Geometry check sheet. Reference: the model listing, model coordinates, mm. A direction names the side the tool comes from. Round coordinates to 2 decimals unless told otherwise and drop trailing zeros. Write each loop counter-clockwise with the first axis right and the second up, starting at its lowest first coordinate (ties: lowest second). Pieces come first, ordered by that corner, then holes.
Item 1: Access from +Z, -Z, +X, -X, +Y, -Y to the whole of each face (thin tool, end or side, straight path). Record for faces 4 (the face through (13.53, -17.05, 0.04)), 5 (the face through (8, 20, 0)), 6 (the face through (-8, 20, 0)).
Item 2: Depth check by flat-ended pin: P1, Ø1.5, axis at y = 23.5, z = -1, coming from the +X side; P2, Ø1, axis at y = -9.5, z = -1.5, coming from the +X side; P3, Ø19, axis at x = 0, y = 0, coming from the -Z side; P4, Ø22, axis at x = 3.5, y = -3.5, coming from the -Z side. Enter the tip coordinate at first touch or a pass-through.
Item 3: Cross-section at D-D (x = -19). Enter the section's corners in (y, z), then the cut area to 3 significant figures.
Item 4: Scan lines: probe 1 along Y at (x, z) = (0, 0); probe 2 along X at (y, z) = (27.5, -0.85); probe 3 along Z at (x, y) = (-0.5, 9). Record each from-to range of solid material in increasing order.
Item 5: Cross-section at C-C (y = 25). Enter the section's corners in (x, z), then the cut area to 3 significant figures.
Item 6: Cross-section at A-A (x = 0). Enter the section's corners in (y, z).
Item 7: Draft check along Z on faces 1 (the face through (-7, 10, -2.5)), 2 (the face through (13.04, 7.41, 0.04)), 3 (the face through (0, -7, 1.5)). Enter one of: pulls with the +Z half, pulls with the -Z half, needs draft (parallel to the pull), parting line crosses it, or undercut.
Item 8: Cross-section at B-B (z = -0.75). Enter the section's corners in (x, y).
from build123d import *

# Parameters (mm, degrees)
F0_R        = 10
F1_DEPTH    = 2.5
F0_R_2      = 6
F2_DEPTH    = 1.5
F3_T1_DEPTH = 15


# Not quite as in the source:
# - a fillet or chamfer that OpenCascade refuses, or shapes differently, is made with other operations: its cross-section is extruded or revolved along the edge and cut away or added


with BuildPart() as f1:
    # F0 (on Top) → F1 (new body, symmetric)
    with BuildSketch(Plane.XY):
        with BuildLine():
            Line((25.9807621135, -15), (29.9807621135, -8.0717967697))
            Line((29.9807621135, -8.0717967697), (14.9886304879, 0.5839144601))
            ThreePointArc((14.9886304879, 0.5839144601), (12.9903810568, 7.5), (8, 12.6885775404))
            Line((8, 12.6885775404), (8, 30))
            Line((8, 30), (-8, 30))
            Line((-8, 30), (-8, 12.6885775404))
            ThreePointArc((-8, 12.6885775404), (-12.9903810568, 7.5), (-14.9886304879, 0.5839144601))
            Line((-14.9886304879, 0.5839144601), (-27.4269246123, -6.5973380009))
            Line((-27.4269246123, -6.5973380009), (-29.9807621135, -8.0717967697))
            Line((-29.9807621135, -8.0717967697), (-21.9807621135, -21.9282032303))
            Line((-21.9807621135, -21.9282032303), (-6.9886304879, -13.2724920005))
            ThreePointArc((-6.9886304879, -13.2724920005), (0, -15), (6.9886304879, -13.2724920005))
            Line((6.9886304879, -13.2724920005), (21.9807621135, -21.9282032303))
            Line((21.9807621135, -21.9282032303), (25.9807621135, -15))
        make_face()
        Circle(F0_R, mode=Mode.SUBTRACT)
    extrude(amount=F1_DEPTH, both=True)

    # F0 (on Top) → F2 (join, symmetric)
    with BuildSketch(Plane.XY):
        Circle(F0_R)
        Circle(F0_R_2, mode=Mode.SUBTRACT)
    extrude(amount=F2_DEPTH, both=True)

    # F3: fillet of radius 2 on 8 edges, made by hand

    # F3_s2 → F3_t1 (cut)
    with BuildSketch(Plane.XY.offset(-7.5)):
        with BuildLine():
            ThreePointArc((-28.9807621135, -9.8038475773), (-29.1805629585, -8.2862094871), (-28.248711306, -7.0717967697))
            Line((-28.248711306, -7.0717967697), (-29.9807621135, -8.0717967697))
            Line((-29.9807621135, -8.0717967697), (-28.9807621135, -9.8038475773))
        make_face()
        with BuildLine():
            ThreePointArc((-20.248711306, -20.9282032303), (-21.7663493962, -21.1280040753), (-22.9807621135, -20.1961524227))
            Line((-22.9807621135, -20.1961524227), (-21.9807621135, -21.9282032303))
            Line((-21.9807621135, -21.9282032303), (-20.248711306, -20.9282032303))
        make_face()
        with BuildLine():
            ThreePointArc((20.248711306, -20.9282032303), (21.7663493962, -21.1280040753), (22.9807621135, -20.1961524227))
            Line((22.9807621135, -20.1961524227), (21.9807621135, -21.9282032303))
            Line((21.9807621135, -21.9282032303), (20.248711306, -20.9282032303))
        make_face()
        with BuildLine():
            ThreePointArc((28.9807621135, -9.8038475773), (29.1805629585, -8.2862094871), (28.248711306, -7.0717967697))
            Line((28.248711306, -7.0717967697), (29.9807621135, -8.0717967697))
            Line((29.9807621135, -8.0717967697), (28.9807621135, -9.8038475773))
        make_face()
        with BuildLine():
            ThreePointArc((8, 28), (7.4142135624, 29.4142135624), (6, 30))
            Line((6, 30), (8, 30))
            Line((8, 30), (8, 28))
        make_face()
        with BuildLine():
            ThreePointArc((-6, 30), (-7.4142135624, 29.4142135624), (-8, 28))
            Line((-8, 28), (-8, 30))
            Line((-8, 30), (-6, 30))
        make_face()
    extrude(amount=F3_T1_DEPTH, mode=Mode.SUBTRACT)

    # F3_s3 → F3_t4 (revolve, cut)
    with BuildSketch(Plane.XZ):
        with BuildLine():
            ThreePointArc((11.7320508076, 2.5), (10.7320508076, 2.2320508076), (10, 1.5))
            Line((10, 1.5), (10, 2.5))
            Line((10, 2.5), (11.7320508076, 2.5))
        make_face()
    revolve(axis=Axis((0, 0, 2.5), (0, 0, 1)), mode=Mode.SUBTRACT)

    # F3_s5 → F3_t6 (revolve, cut)
    with BuildSketch(Plane.XZ):
        with BuildLine():
            ThreePointArc((11.7320508076, -2.5), (10.7320508076, -2.2320508076), (10, -1.5))
            Line((10, -1.5), (10, -2.5))
            Line((10, -2.5), (11.7320508076, -2.5))
        make_face()
    revolve(axis=Axis((0, 0, -2.5), (0, 0, 1)), mode=Mode.SUBTRACT)


solid = f1.part
Resolved:
1. face 4: +Z, -Z, -Y
1. face 5: +Z, -Z, +X, +Y
1. face 6: +Z, -Z, -X, +Y
2. P1: stops at x = 8
2. P2: stops at x = 29.24
2. P3: stops at z = -1.5
2. P4: stops at z = -2.5
3. outline: (-20.21, -2.5) - (-1.73, -2.5) - (-1.73, 2.5) - (-20.21, 2.5) - close
3. area: 92.4 mm2
4. probe 1: y = -15 to -6, 6 to 30
4. probe 2: x = -8 to 8
4. probe 3: z = -1.5 to 1.5
5. outline: (-8, -2.5) - (8, -2.5) - (8, 2.5) - (-8, 2.5) - close
5. area: 80.0 mm2
6. outline: (-15, -2.5) - (-11.73, -2.5) arc R2 ccw to (-10, -1.5) - (-6, -1.5) - (-6, 1.5) - (-10, 1.5) arc R2 ccw to (-11.73, 2.5) - (-15, 2.5) - close; (6, -1.5) - (10, -1.5) arc R2 ccw to (11.73, -2.5) - (30, -2.5) - (30, 2.5) - (11.73, 2.5) arc R2 ccw to (10, 1.5) - (6, 1.5) - close
7. face 1: pulls with the -Z half
7. face 2: needs draft
7. face 3: pulls with the +Z half
8. outline: (-28.98, -9.8) - (-22.98, -20.2) arc R2 ccw to (-20.25, -20.93) - (-6.99, -13.27) arc R15 ccw to (6.99, -13.27) - (20.25, -20.93) arc R2 ccw to (22.98, -20.2) - (28.98, -9.8) arc R2 ccw to (28.25, -7.07) - (14.99, 0.58) arc R15 ccw to (8, 12.69) - (8, 28) arc R2 ccw to (6, 30) - (-6, 30) arc R2 ccw to (-8, 28) - (-8, 12.69) arc R15 ccw to (-14.99, 0.58) - (-28.25, -7.07) arc R2 ccw to start; hole circle Ø12 at (0, 0)
